Geometry: see drawing. Coordinates: mm, zero at the bounding-box minimum. Give positions to 0.01 mm unless a question says otherwise; leave off trailing zeros. Write each loop counter-clockwise with the first axis right and the second up, starting at its lowest first coordinate (ties: lowest second). Pieces come first, ordered by that corner, then holes. Notation, with made-up numbers: (11, 25) -> (23, 25) arc R38 ccw to (23, 63) -> close; hole circle Ø3 at (41, 61). An arc over 180 degrees is marked (long way). Use CSV: the item, a comma, the result in double quotes. Start each with the question number.
1) Section A-A (x = 10). Output: boundary loops of the cut face in (y, z) (3 decimals).
2) Section C-C (y = 10). Output: boundary loops of the cut face in (x, z) (1 decimal), plus the area to 3 significant figures.
3) Section B-B (z = 2.5). Output: boundary loops of the cut face in (x, y).
4) Material intervals for line 1 (Y direction, x = 10, z = 2.35); line 2 (X direction, y = 8.25, z = 1.05); line 3 (X direction, y = 10, z = 2.35), sorted ascending. Write a range as [from, to].
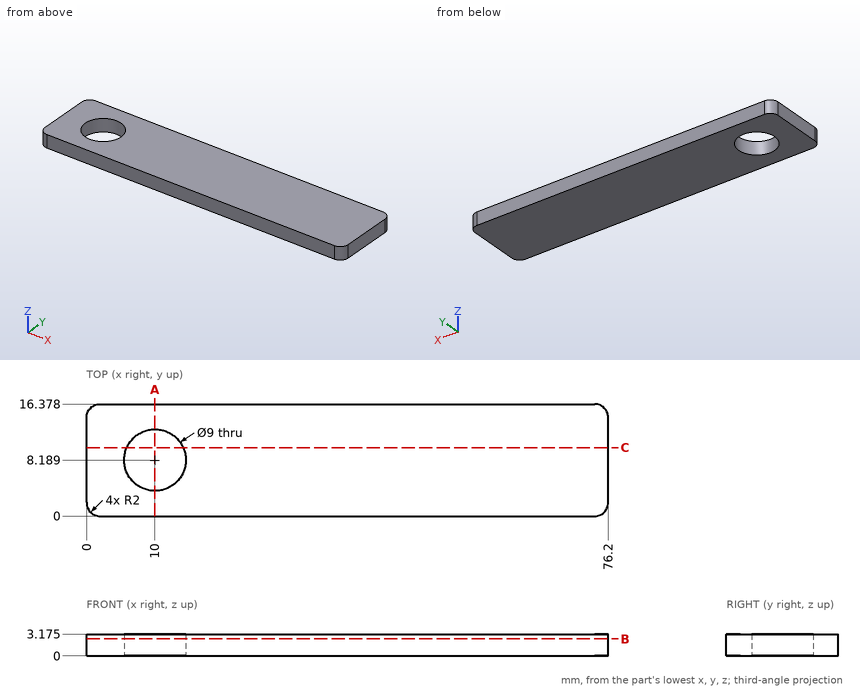
Answers follow:
1,outline,"(0, 0) -> (3.689, 0) -> (3.689, 3.175) -> (0, 3.175) -> close; (12.689, 0) -> (16.378, 0) -> (16.378, 3.175) -> (12.689, 3.175) -> close"
2,outline,"(0, 0) -> (5.9, 0) -> (5.9, 3.2) -> (0, 3.2) -> close; (14.1, 0) -> (76.2, 0) -> (76.2, 3.2) -> (14.1, 3.2) -> close"
2,area,"216 mm^2"
3,outline,"(0, 2) arc R2 ccw to (2, 0) -> (74.2, 0) arc R2 ccw to (76.2, 2) -> (76.2, 14.38) arc R2 ccw to (74.2, 16.38) -> (2, 16.38) arc R2 ccw to (0, 14.38) -> close; hole circle Ø9 at (10, 8.19)"
4,line 1,"y = [0, 3.69], [12.69, 16.38]"
4,line 2,"x = [0, 5.5], [14.5, 76.2]"
4,line 3,"x = [0, 5.88], [14.12, 76.2]"
